Verification items for the finished model (mm, model axes). Face numbers are marked on the shaded views. A direction names the side the tool comes from. Round coordinates to 2 decimals unless told otherwise and drop trailing zeros. Order: outer loops, then holes, each group sorted by start corner. A loop starts at its lowest first (then second) coordinate and runs counter-clockwise, first axis right, second up. Notation, with made-up numbers: (-35.5, -7.5) -> (-26.5, -7.5) arc R17 cw to (-26.5, 22.5) -> close; hole circle Ø6 at (70, -28.5). An arc over 180 degrees is marked (long way). Put each result on its own line as item: value.
from build123d import *

# Parameters (mm, degrees)
PAD_DEPTH    = 3.2
SKETCH001_W  = 11
SKETCH001_H  = 11
PAD001_DEPTH = 1


with BuildPart() as part:
    # Sketch → Pad (new body)
    with BuildSketch(Plane.XY):
        with BuildLine():
            Line((-1, 0), (-6.9, 0))
            ThreePointArc((-7.9, 1), (-7.607107, 0.292893), (-6.9, 0))
            Line((-7.9, 1), (-7.9, 6.9))
            ThreePointArc((-6.9, 7.9), (-7.607107, 7.607107), (-7.9, 6.9))
            Line((-6.9, 7.9), (-1, 7.9))
            ThreePointArc((0, 6.9), (-0.292893, 7.607107), (-1, 7.9))
            Line((0, 6.9), (0, 1))
            ThreePointArc((-1, 0), (-0.292893, 0.292893), (0, 1))
        make_face()
    extrude(amount=PAD_DEPTH)

    # Sketch001 (on DatumPlane) → Pad001 (join)
    with BuildSketch(Plane(origin=(0, 0, 0), x_dir=(1, 0, 0), z_dir=(0, 0, -1))):
        with Locations((-3.95, -3.95)):
            Rectangle(SKETCH001_W, SKETCH001_H)
    extrude(amount=PAD001_DEPTH)


solid = part.part
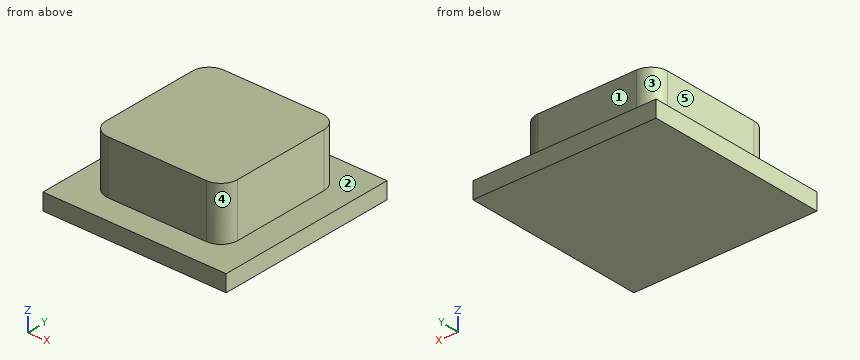
Item 1: Section check B-B on z = 1. Record the boundary of the cut face in (x, y).
Check sheet entries:
outline: (-7.9, 1) arc R1 ccw to (-6.9, 0) -> (-1, 0) arc R1 ccw to (0, 1) -> (0, 6.9) arc R1 ccw to (-1, 7.9) -> (-6.9, 7.9) arc R1 ccw to (-7.9, 6.9) -> close
Item 2: Section check D-D on y = 9.25. Record the boundary of the cut face in (x, z), then the cut area to 3 significant figures.
Check sheet entries:
outline: (-9.45, -1) -> (1.55, -1) -> (1.55, 0) -> (-9.45, 0) -> close
area: 11.0 mm^2
Item 3: Material ranges on L1, parallel to Y at x = -6.25, z = 2.15; L2, parallel to Z at x = -8.5, y = 7.5; L3, parallel to X at y = 2, z = 0.95, recorded low to high. Write a range as [from, to].
Check sheet entries:
L1: y = [0, 7.9]
L2: z = [-1, 0]
L3: x = [-7.9, 0]
Item 4: Gauge pin test, flat ends, axial feed: pin 1 Ø1.5 at (x, z) = (-2.5, 1) entering from +Y; pin 2 Ø1 at (y, z) = (5, 2) entering from -X; pin 3 Ø1.6 at (y, z) = (3.5, 1.5) entering from +X. Record the tip position at first contact, or that the pin passes through.
Check sheet entries:
pin 1: stops at y = 7.9
pin 2: stops at x = -7.9
pin 3: stops at x = 0
Item 5: Tool access check on the marked faces 1, 2, 3, 4 and 5. Record the directions out of +Z, -Z, +X, -X, +Y, -Y that give a thin tool (end or side, any length) a straight path to the whole face; none if there is none.
Check sheet entries:
face 1: +Z, +X, -X, +Y
face 2: +Z
face 3: +Z, -X, +Y
face 4: +Z, +X, -Y
face 5: +Z, -X, +Y, -Y
Item 6: Section check C-C on x = 0.5. Record the boundary of the cut face in (y, z).
Check sheet entries:
outline: (-1.55, -1) -> (9.45, -1) -> (9.45, 0) -> (-1.55, 0) -> close
Item 7: Section check A-A on y = 6.25. Record the boundary of the cut face in (x, z).
Check sheet entries:
outline: (-9.45, -1) -> (1.55, -1) -> (1.55, 0) -> (0, 0) -> (0, 3.2) -> (-7.9, 3.2) -> (-7.9, 0) -> (-9.45, 0) -> close
